Read the model definition and answer for the solid it produces. Units are mm, in the model's axes. A direction names the side the tool comes from. Round coordinates to 2 decimals unless told otherwise and drop trailing zeros. Order: outer loops, then holes, each group sorted by start corner. A loop starts at its lowest first (then second) coordinate and runs counter-clockwise, first axis right, second up. Notation, with made-up numbers: (-35.5, -5) - (-16.5, -5) arc R7 ccw to (-16.5, 5) - close; hole circle Ø8 at (-33, 46). An arc over 180 degrees is marked (long way). Put each result on its own line as item: value. Start each with the question number.
Q1. Find the intervals of material crossed by line 1 along Y through (x, z) = (0, 3.9); line 2 along X through (y, z) = (16.15, 0); line 3 along Y through (x, z) = (-0.25, -1.75), in increasing order. Write a range as from..to.
Q2. Section B-B on z = 0 is taken. Give the vertices of the cut face in (x, y), then the cut area to 3 significant figures.
Q3. Each of these flat-tipped pins is pushed along its axis until it touches: pin 1 Ø4 at (x, z) = (0, 0) entering from -Y; pin 2 Ø1.5 at (x, z) = (-0.5, 0) entering from +Y. Where does it stop, or does it pass through?
Q4. Section C-C on y = 5.25 is taken. Give the vertices of the cut face in (x, z), then the cut area to 3 significant figures.
Q5. Section A-A on x = 0 is taken. Give the vertices of the cut face in (y, z), then the cut area to 3 significant figures.
Q6. For a pull along X with two mould halves and no side action, classify faces 4 (the face through (0, 10, 0)), 5 (the face through (-1.2, 20, -1.2)), 6 (the face through (2.634, 9.86, -4.132)) as pulls with the +X half, pulls with the -X half, needs draft (parallel to the pull), parting line crosses it, or undercut.
Q7. Section D-D on y = 8.25 is taken. Give the vertices of the cut face in (x, z), then the cut area to 3 significant figures.
Q8. Which of the six approach directions +Z, -Z, +X, -X, +Y, -Y give full straight-line access (tool end or side, diameter ignored) to faces 1 (the face through (-1.5, 17.54, -0.07)), 2 (the face through (-3.4, 4.9, 0.1)), 3 (the face through (-0.54, 2.56, 3.58))?
from build123d import *

# Parameters (mm, degrees)
SKETCH1_R               = 4.9
BOSS_EXTRUDE1_DEPTH     = 20
SKETCH2_R               = 1.5
CUT_EXTRUDE1_DEPTH      = 5
SKETCH3_R               = 3.4
CUT_EXTRUDE2_DEPTH      = 10
SKETCH4_R               = 2.5
CUT_EXTRUDE3_DEPTH      = 5.9
CUT_EXTRUDE3_DEPTH_BACK = 5.9


with BuildPart() as part:
    # Sketch1 → Boss-Extrude1 (new body)
    with BuildSketch(Plane(origin=(0, 0, 0), x_dir=(1, 0, 0), z_dir=(0, 1, 0))):
        Circle(SKETCH1_R)
    extrude(amount=BOSS_EXTRUDE1_DEPTH)

    # Sketch2 → Cut-Extrude1 (cut)
    with BuildSketch(Plane(origin=(0, 20, 0), x_dir=(1, 0, 0), z_dir=(0, 1, 0))):
        Circle(SKETCH2_R)
    extrude(amount=-CUT_EXTRUDE1_DEPTH, mode=Mode.SUBTRACT)

    # Sketch3 → Cut-Extrude2 (cut)
    with BuildSketch(Plane.XZ):
        Circle(SKETCH3_R)
    extrude(amount=-CUT_EXTRUDE2_DEPTH, mode=Mode.SUBTRACT)

    # Sketch4 → Cut-Extrude3 (cut, two sides)
    with BuildSketch(Plane.XY) as cut_extrude3_sk:
        with Locations((0, 5)):
            Circle(SKETCH4_R)
    extrude(amount=CUT_EXTRUDE3_DEPTH, mode=Mode.SUBTRACT)
    extrude(cut_extrude3_sk.sketch, amount=-CUT_EXTRUDE3_DEPTH_BACK, mode=Mode.SUBTRACT)


solid = part.part
Findings:
1. line 1: 0..2.5, 7.5..20
1. line 2: -4.9..-1.5, 1.5..4.9
1. line 3: 10..20
2. outline: (-4.9, 0) - (-3.4, 0) - (-3.4, 10) - (3.4, 10) - (3.4, 0) - (4.9, 0) - (4.9, 20) - (1.5, 20) - (1.5, 15) - (-1.5, 15) - (-1.5, 20) - (-4.9, 20) - close
2. area: 113 mm2
3. pin 1: y = 10
3. pin 2: y = 15
4. outline: (-2.49, -4.22) - (-2.49, -2.32) arc R3.4 cw to (-2.49, 2.32) - (-2.49, 4.22) arc R4.9 ccw to start; (2.49, -4.22) arc R4.9 ccw to (2.49, 4.22) - (2.49, 2.32) arc R3.4 cw to (2.49, -2.32) - close
4. area: 23.0 mm2
5. outline: (0, -4.9) - (2.5, -4.9) - (2.5, -3.4) - (0, -3.4) - close; (0, 3.4) - (2.5, 3.4) - (2.5, 4.9) - (0, 4.9) - close; (7.5, -4.9) - (20, -4.9) - (20, -1.5) - (15, -1.5) - (15, 1.5) - (20, 1.5) - (20, 4.9) - (7.5, 4.9) - (7.5, 3.4) - (10, 3.4) - (10, -3.4) - (7.5, -3.4) - close
5. area: 98.0 mm2
6. face 4: undercut
6. face 5: needs draft
6. face 6: parting line crosses it
7. outline: circle Ø9.8 at (0, 0); hole circle Ø6.8 at (0, 0)
7. area: 39.1 mm2
8. face 1: +Y
8. face 2: -Y
8. face 3: +Z, -Z
